The figure shows three views and two pictorial views of one solid part (mm, origin at its lowest corner). Answer the questions. Coordinates: 2 decimals unless noted, no trailing zeros. Order: outer loops, then holes, each group sorted by start corner. A loop starts at its lowest first (then second) coordinate and runs counter-clockwise, first axis right, second up. Notation, with made-up numbers: (13, -9.5) - (49, -9.5) arc R12 ccw to (49, 4.5) - close; hole circle Ø11 at (55, -1.5). An arc over 180 degrees is marked (long way). Answer as a JSON object with one key per item and string values. Group by question number.
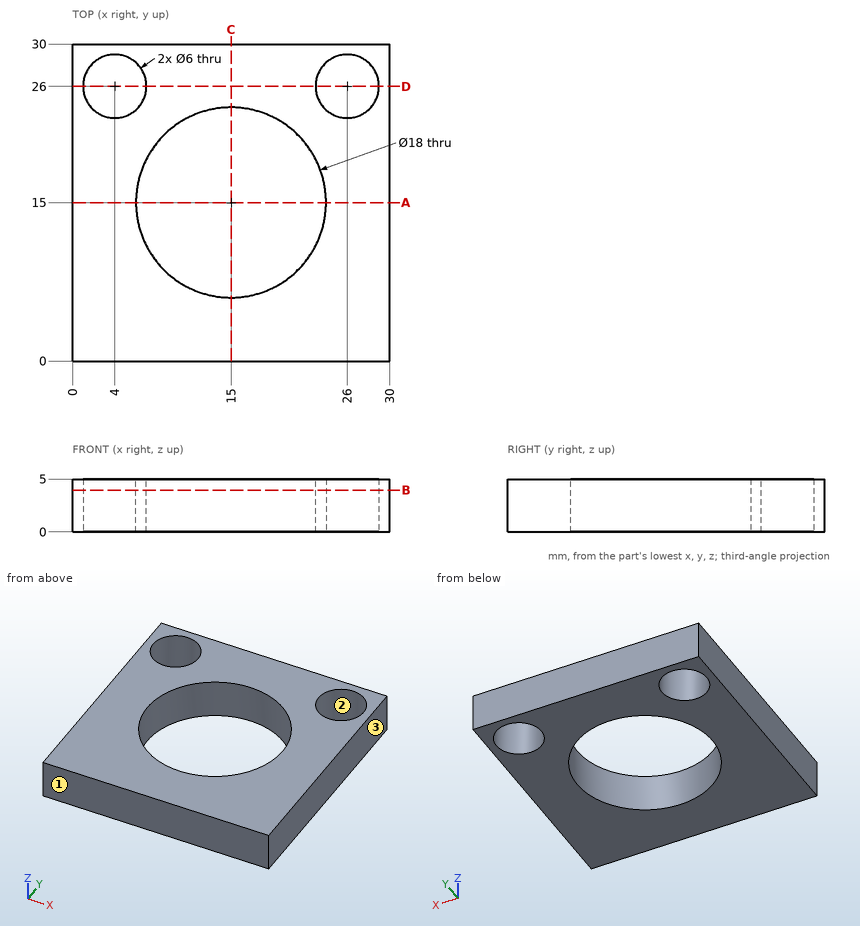
1. Straight lines are drawn through the part: L1, parallel to Y at x = 15, z = 3.4; L2, parallel to Y at x = 4, z = 3.85; L3, parallel to X at y = 9, z = 3.55. For each, find the intervals that lie inside material, in ascending order.
2. A cutting plane is placed at B-B on z = 3.95. Write down the section's boundary in (x, y).
3. A cutting plane is placed at A-A on y = 15. Write down the section's boundary in (x, z), and give its area (3 significant figures).
4. Given pin 1 (1.5 mm diameter, centred on x = 21, y = 18.5, fed in from +Z), flat-ended and moving along its own axis, determine where the tip first touches the part or whether it passes through.
5. For a pull along Y with two mould halves and no side action, classify the marked faces 1, 2 and 3 as pulls with the +Y half, pulls with the -Y half, needs draft (parallel to the pull), parting line crosses it, or undercut.
6. A cutting plane is placed at D-D on y = 26. Write down the section's boundary in (x, z), and give its area (3 significant figures).
Derived:
{
 "1": {"L1": "y = 0 to 6, 24 to 30", "L2": "y = 0 to 23, 29 to 30", "L3": "x = 0 to 8.29, 21.71 to 30"},
 "2": {"outline": "(0, 0) - (30, 0) - (30, 30) - (0, 30) - close; hole circle Ø6 at (4, 26); hole circle Ø18 at (15, 15); hole circle Ø6 at (26, 26)"},
 "3": {"outline": "(0, 0) - (6, 0) - (6, 5) - (0, 5) - close; (24, 0) - (30, 0) - (30, 5) - (24, 5) - close", "area": "60.0 mm2"},
 "4": {"pin 1": "passes through"},
 "5": {"face 1": "pulls with the -Y half", "face 2": "undercut", "face 3": "needs draft"},
 "6": {"outline": "(0, 0) - (1, 0) - (1, 5) - (0, 5) - close; (7, 0) - (23, 0) - (23, 5) - (7, 5) - close; (29, 0) - (30, 0) - (30, 5) - (29, 5) - close", "area": "90.0 mm2"}
}
